For this review, take the finished solid that the model builds, in its own axes (mm). A direction names the side the tool comes from. Give positions to 0.01 mm unless a question says otherwise; leave off trailing zeros. Loops run counter-clockwise (first coordinate to the right, second up) from the corner with the lowest first, then second, coordinate; pieces in that order, holes last. Notation, with made-up numbers: (61.25, -39) -> (109.25, -39) arc R18 ccw to (109.25, -25) -> close; hole circle Ø1 at (-10, 51). An arc over 180 degrees is marked (long way). Answer as CSV lines item,"result". Start each with the question number.
Item 1: Add section B-B on x = 0. State the section outline as (y, z) points, plus the area to 3 significant figures.
Item 2: Add section D-D on x = -14. State the section outline as (y, z) points.
Item 3: Machinability: for faces 5 (the face through (0, 6, 4)), 6 (the face through (-14.9, -1.4, 5)), which of the approach directions +Z, -Z, +X, -X, +Y, -Y give a long, thin tool a straight path to every point of the face, cutting with its end or side? Answer none if there is none.
Item 4: The part is to be moulded in two halves that separate along Y. For faces 1 (the face through (-17.43, -5.4, 2.54)), 2 (the face through (13.1, -1.4, 5)), 3 (the face through (-15.5, 0.07, 2.54)), 4 (the face through (-17.43, 5.4, 2.54)), say which applies: +Y half, -Y half, draft (parallel to the pull), parting line (faces both ways), or undercut.
Item 5: Add section C-C on z = 6.5. State the section outline as (x, y) points, plus the area to 3 significant figures.
Item 6: For L1, parallel to Y at x = -14, z = 1.8; L2, parallel to Z at x = 12, y = -4; L3, parallel to Y at x = 0, z = 5.5, list the stretches that pass through material, from the lowest coordinate up. Write a range as from..to.
Item 7: Add section A-A on y = 0. State the section outline as (x, z) points.
Item 8: Clearance check with flat-ended pins moving along their axes: P1, Ø6.5, axis at x = 16, y = 1.5, coming from the +Z side; P2, Ø4, axis at y = 1, z = 6, coming from the +X side; P3, Ø2, axis at x = -11, z = 6.5, coming from the -Y side. State where each tip first meets the part, or that it passes through.
```python
from build123d import *

# Parameters (mm, degrees)
ESQUISSE1_W             = 36
ESQUISSE1_H             = 12
ESQUISSE1_R             = 3
BOSS_EXTRU_1_DEPTH      = 10
ESQUISSE2_R             = 1.5
ENL_V_MAT_EXTRU_1_DEPTH = 22.44761059
ESQUISSE3_OUTSIDE_W     = 45.848
ESQUISSE3_OUTSIDE_H     = 19.848
ENL_V_MAT_EXTRU_2_DEPTH = 24.832750576
CONG_1_R                = 2


with BuildPart() as part:
    # Esquisse1 → Boss.-Extru.1 (new body)
    with BuildSketch(Plane.XY):
        Rectangle(ESQUISSE1_W, ESQUISSE1_H)
        Circle(ESQUISSE1_R, mode=Mode.SUBTRACT)
    extrude(amount=BOSS_EXTRU_1_DEPTH)

    # Esquisse2 → Enlèv. mat.-Extru.1 (cut, through all)
    with BuildSketch(Plane.XY.offset(10)):
        with Locations((-14, 0)):
            Circle(ESQUISSE2_R)
        with Locations((14, 0)):
            Circle(ESQUISSE2_R)
    extrude(amount=-ENL_V_MAT_EXTRU_1_DEPTH, mode=Mode.SUBTRACT)

    # Esquisse3 outside → Enlèv. mat.-Extru.2 (cut, through all)
    with BuildSketch(Plane.XZ.offset(6)):
        with Locations((0, 5)):
            Rectangle(ESQUISSE3_OUTSIDE_W, ESQUISSE3_OUTSIDE_H)
        Polygon((-18, 0), (-18, 5), (-10, 5), (-7.113248654, 10), (7.113248654, 10), (10, 5), (18, 5), (18, 0), align=None, mode=Mode.SUBTRACT)
    extrude(amount=-ENL_V_MAT_EXTRU_2_DEPTH, mode=Mode.SUBTRACT)

    # Congé1
    cong_1_edges = [part.edges().sort_by_distance(p)[0] for p in [
        (-18, 6, 2.5),
        (18, 6, 2.5),
        (18, -6, 2.5),
        (-18, -6, 2.5),
    ]]
    fillet(cong_1_edges, radius=CONG_1_R)


solid = part.part
```
Computed values:
1,outline,"(-6, 0) -> (-3, 0) -> (-3, 10) -> (-6, 10) -> close; (3, 0) -> (6, 0) -> (6, 10) -> (3, 10) -> close"
1,area,"60.0 mm²"
2,outline,"(-6, 0) -> (-1.5, 0) -> (-1.5, 5) -> (-6, 5) -> close; (1.5, 0) -> (6, 0) -> (6, 5) -> (1.5, 5) -> close"
3,face 5,"+Z, -Z, +X, -X, +Y"
3,face 6,"+Z, -X, +Y, -Y"
4,face 1,"-Y half"
4,face 2,"draft"
4,face 3,"undercut"
4,face 4,"+Y half"
5,outline,"(-9.13, -6) -> (9.13, -6) -> (9.13, 6) -> (-9.13, 6) -> close; hole circle Ø6 at (0, 0)"
5,area,"191 mm²"
6,L1,"-6..-1.5, 1.5..6"
6,L2,"0..5"
6,L3,"-6..-3, 3..6"
7,outline,"(-18, 0) -> (-15.5, 0) -> (-15.5, 5) -> (-18, 5) -> close; (-12.5, 0) -> (-3, 0) -> (-3, 10) -> (-7.11, 10) -> (-10, 5) -> (-12.5, 5) -> close; (3, 0) -> (12.5, 0) -> (12.5, 5) -> (10, 5) -> (7.11, 10) -> (3, 10) -> close; (15.5, 0) -> (18, 0) -> (18, 5) -> (15.5, 5) -> close"
8,P1,"z = 5"
8,P2,"x = 18"
8,P3,"through"
